from build123d import *

# Parameters (mm, degrees)
SKETCH_1_W             = 25
SKETCH_1_H             = 25
SKETCH_1_W_2           = 19
SKETCH_1_H_2           = 19
EXTRUDE_1_DEPTH        = 685.5
HOLE_WIZARD_6_0_6_1_D  = 6
CUT_EXTRUDE_1_REACH    = 688.411
SKETCH_5_R             = 6
PATTERN_LINEAR_1_COUNT = 2
PATTERN_LINEAR_1_PITCH = 650.3


with BuildPart() as part:
    # 草图1 → 拉伸1 (new body)
    with BuildSketch(Plane.XY):
        with Locations((12.5, -12.5)):
            Rectangle(SKETCH_1_W, SKETCH_1_H)
        with Locations((12.5, -12.5)):
            Rectangle(SKETCH_1_W_2, SKETCH_1_H_2, mode=Mode.SUBTRACT)
    extrude(amount=EXTRUDE_1_DEPTH)

    # Ø6.0 (6) 直径孔1 (through all)
    with Locations(Plane(origin=(25, 0, 0), x_dir=(0, 0, -1), z_dir=(1, 0, 0))):
        with Locations((-667.65, -12.5)):
            hole_wizard_6_0_6_1 = Hole(HOLE_WIZARD_6_0_6_1_D / 2)

    # 草图5 → 切除-拉伸1 (cut, up to next)
    with BuildSketch(Plane.ZY, mode=Mode.PRIVATE) as cut_extrude_1_sk1:
        with Locations(Location((667.65, -12.5, 0), (0, 0, 270))):
            Circle(SKETCH_5_R)
    cut_extrude_1_tool1 = extrude(cut_extrude_1_sk1.sketch, amount=-CUT_EXTRUDE_1_REACH, mode=Mode.PRIVATE) & part.part
    cut_extrude_1 = cut_extrude_1_tool1.solids().sort_by_distance((0, -12.5, 667.65))[0]
    add(cut_extrude_1, mode=Mode.SUBTRACT)

    # 阵列(线性)1: Ø6.0 (6) 直径孔1, 切除-拉伸1 ×2
    with Locations(*[(0, 0, -i * PATTERN_LINEAR_1_PITCH) for i in range(1, PATTERN_LINEAR_1_COUNT)]):
        add(hole_wizard_6_0_6_1, mode=Mode.SUBTRACT)
        add(cut_extrude_1, mode=Mode.SUBTRACT)


solid = part.part
For this review, take the finished solid that the model builds, in its own axes (mm). A direction names the side the tool comes from. Give positions to 0.01 mm unless a question says otherwise; leave off trailing zeros. Order: outer loops, then holes, each group sorted by start corner. A loop starts at its lowest first (then second) coordinate and runs counter-clockwise, first axis right, second up. Notation, with made-up numbers: (-11.75, 71.5) -> (37.25, 71.5) arc R22 cw to (37.25, 101.5) -> close; hole circle Ø5 at (39, -22). An arc over 180 degrees is marked (long way). Write item = value, one per line.
1) For faces 1 (the face through (1.48, -18.04, 15.05)), 2 (the face through (3, -13, 338)), 3 (the face through (12, -25, 338)), list the 3-axis set-ups (+Z, -Z, +X, -X, +Y, -Y) from which the entire face can be reached by the end or side of a thin tool; tool diameter is ignored.
Findings:
face_1 = -X
face_2 = +Z, -Z
face_3 = +Z, -Z, +X, -X, -Y
2) We need section A-A, the plane x = 13. Give the boundary of the cut face in (y, z).
Findings:
outline = (-25, 0) -> (-22, 0) -> (-22, 685.5) -> (-25, 685.5) -> close; (-3, 0) -> (0, 0) -> (0, 685.5) -> (-3, 685.5) -> close
3) Insertion check: pin 1 (9.5 mm diameter, centred on y = -12.5, z = 17.35, fed in from -X); pin 2 (3.5 mm diameter, centred on y = -12.5, z = 667.65, fed in from +X). Each pin has a flat end and moves straight along its axis. Give the tip position at first contact, or say it passes through.
Findings:
pin_1 = 22
pin_2 = through
4) We need section B-B, the plane z = 628. Give the boundary of the cut face in (x, y).
Findings:
outline = (0, -25) -> (25, -25) -> (25, 0) -> (0, 0) -> close; hole (3, -22) -> (22, -22) -> (22, -3) -> (3, -3) -> close
5) To check wall thickness, follow L1, parallel to Z at x = 1.65, y = -12.5; L2, parallel to Y at x = 18, z = 348.5; L3, parallel to X at y = -13.5, z = 148.5. State the ranges of each line that lie inside material, in increasing order. Write a range as from..to.
Findings:
L1 = 0..11.35, 23.35..661.65, 673.65..685.5
L2 = -25..-22, -3..0
L3 = 0..3, 22..25
6) Draft analysis for pull direction X (two halves, no side actions). For faces 4 (the face through (22, -13, 338)), 5 (the face through (1.48, -11.72, 673.6)), 6 (the face through (12, -3, 338)), 7 (the face through (0, -13, 338)), state which applies: pulls with the +X half, pulls with the -X half, needs draft (parallel to the pull), parting line crosses it, or undercut.
Findings:
face_4 = undercut
face_5 = needs draft
face_6 = undercut
face_7 = pulls with the -X half
